Could you check a few things on this model? Use its own coordinates, in mm. A direction names the side the tool comes from. Coordinates: 2 decimals unless noted, no trailing zeros. Loops run counter-clockwise (first coordinate to the right, second up) from the corner with the lowest first, then second, coordinate; pieces in that order, holes last.
Autodesk Inventor part; units mm, degrees
ref_plane "YZ Plane" through (0, 0, 0) normal (1, 0, 0) x (0, 1, 0)
ref_plane "XZ Plane" through (0, 0, 0) normal (0, 1, 0) x (-1, 0, 0)
ref_plane "XY Plane" through (0, 0, 0) normal (0, 0, 1) x (1, 0, 0)
sketch "Sketch1" plane through (0, 0, 0) normal (0, 0, 1) x (1, 0, 0)
  line L0 (-11, -22.75) -> (11, -22.75)
  line L1 (11, -22.75) -> (11, 22.75)
  line L2 (11, 22.75) -> (-11, 22.75)
  line L3 (-11, 22.75) -> (-11, -22.75)
  circle A0 centre (-8, 0) radius 2.25
  line L4 (-5, 22.75) -> (-5, -22.75) construction
  line L5 (5, 22.75) -> (5, -22.75) construction
  line L6 (0, 22.75) -> (0, -22.75) construction
  circle A1 centre (-8, 19.75) radius 2.25
  circle A2 centre (-8, -19.75) radius 2.25
  circle A3 centre (8, -19.75) radius 2.25
  circle A4 centre (8, 0) radius 2.25
  circle A5 centre (8, 19.75) radius 2.25
  line L7 (-11, 0) -> (11, 0) construction
  line L8 (-11, 22.75) -> (11, 22.75)
  line L9 (11, 22.75) -> (11, 16.75)
  line L10 (11, 16.75) -> (-11, 16.75)
  line L11 (-11, 16.75) -> (-11, 22.75)
  line L12 (-11, 3) -> (11, 3)
  line L13 (11, 3) -> (11, -3)
  line L14 (11, -3) -> (-11, -3)
  line L15 (-11, -3) -> (-11, 3)
  line L16 (-11, -22.75) -> (11, -22.75)
  line L17 (11, -22.75) -> (11, -16.75)
  line L18 (11, -16.75) -> (-11, -16.75)
  line L19 (-11, -16.75) -> (-11, -22.75)
  point P0 (0, 0)
  dimension "d0" = 4.5
  dimension "d1" = 3
  dimension "d2" = 3
  dimension "d3" = 10
  dimension "d5" = 4.5
  dimension "d6" = 3
  dimension "d7" = 3
  dimension "d8" = 4.5
  dimension "d9" = 3
  dimension "d10" = 3
  dimension "d11" = 3
  dimension "d14" = 22
  dimension "d15" = 3
  dimension "d16" = 3
  dimension "d17" = 3
  dimension "d18" = 3
extrude "Extrusion1" add sketch "Sketch1" along normal blind 0.6
extrude "Extrusion2" add sketch "Sketch1" along normal blind 1.8 contours L3 L18 L1 L0 | L3 L12 L1 L14 | L3 L2 L1 L10
properties part number "FoldLink" material "Rubber, Silicone"
(1) Imagine slicing it at D-D, the plane x = 5. Write out the boundary of the cut face in (y, z), and give its area (3 significant figures).
Answers:
outline: (-22.75, 0) - (22.75, 0) - (22.75, 1.8) - (16.75, 1.8) - (16.75, 0.6) - (3, 0.6) - (3, 1.8) - (-3, 1.8) - (-3, 0.6) - (-16.75, 0.6) - (-16.75, 1.8) - (-22.75, 1.8) - close
area: 48.9 mm2
(2) Imagine slicing it at C-C, the plane y = 0. Write out the boundary of the cut face in (x, z), and give its area (3 significant figures).
Answers:
outline: (-11, 0) - (-10.25, 0) - (-10.25, 1.8) - (-11, 1.8) - close; (-5.75, 0) - (5.75, 0) - (5.75, 1.8) - (-5.75, 1.8) - close; (10.25, 0) - (11, 0) - (11, 1.8) - (10.25, 1.8) - close
area: 23.4 mm2
(3) For pin 1 (12 mm diameter, centred on x = 2.5, y = 10, fed in from +Z), with a flat end and sliding along its axis, tell me the tip position at first contact or that it passes through.
Answers:
pin 1: stops at z = 0.6
(4) Which directions (+Z, -Z, +X, -X, +Y, -Y) give clear straight access to the entire face, cutting with the end or side of a thin tool? Please do faces 5 (the face through (5.752, -0.099, 0.887)), 6 (the face through (0, -16.75, 1)).
Answers:
face 5: +Z, -Z
face 6: +Z, +X, -X
(5) We'd pull the mould along X, two halves only. Please class faces 1 (the face through (8, 22, 1)), 2 (the face through (0, -3, 1)), 3 (the face through (-11, 0, 1)), 4 (the face through (11, 0, 1)): +X half, -X half, draft (parallel to the pull), parting line (faces both ways), or undercut.
Answers:
face 1: undercut
face 2: draft
face 3: -X half
face 4: +X half
(6) I need wall thicknesses on probe 1 along Y at (x, z) = (8, 0.55); probe 2 along Y at (x, z) = (8, 1.2); probe 3 along Y at (x, z) = (1, 1.45). Which ranges of each line are inside material? Lowest first, please.
Answers:
probe 1: y = -22.75 to -22, -17.5 to -2.25, 2.25 to 17.5, 22 to 22.75
probe 2: y = -22.75 to -22, -17.5 to -16.75, -3 to -2.25, 2.25 to 3, 16.75 to 17.5, 22 to 22.75
probe 3: y = -22.75 to -16.75, -3 to 3, 16.75 to 22.75
(7) Imagine slicing it at B-B, the plane x = -8. Write out the boundary of the cut face in (y, z).
Answers:
outline: (-22.75, 0) - (-22, 0) - (-22, 1.8) - (-22.75, 1.8) - close; (-17.5, 0) - (-2.25, 0) - (-2.25, 1.8) - (-3, 1.8) - (-3, 0.6) - (-16.75, 0.6) - (-16.75, 1.8) - (-17.5, 1.8) - close; (2.25, 0) - (17.5, 0) - (17.5, 1.8) - (16.75, 1.8) - (16.75, 0.6) - (3, 0.6) - (3, 1.8) - (2.25, 1.8) - close; (22, 0) - (22.75, 0) - (22.75, 1.8) - (22, 1.8) - close
(8) Imagine slicing it at A-A, the plane z = 1.45. State how many separate pieces and enclosed holes the cut face has, and give its area (3 significant figures).
Answers:
separate pieces: 3
enclosed holes: 6
area: 301 mm2
